Work out the finished part from the listing and answer in its coordinate system (mm). Face numbers are marked on the shaded views. A direction names the side the tool comes from. Round coordinates to 2 decimals unless told otherwise and drop trailing zeros. Order: outer loops, then holes, each group sorted by start corner. A loop starts at its lowest first (then second) coordinate and runs counter-clockwise, first axis right, second up. Notation, with made-up numbers: (12, 56) - (68, 56) arc R16 ccw to (68, 84) - close; hole circle Ø6 at (55.25, -28.75). An arc over 180 degrees is marked (long way). Use one line per item in the form item = value. Start each with the question number.
Q1. The part is cut by section D-D on z = -8.5. Determine the outline of the cut face in (x, y).
Q2. The part is cut by section C-C on x = 33.5. Determine the outline of the cut face in (y, z).
Q3. The part is cut by section B-B on z = -27.5. Determine the outline of the cut face in (x, y), plus the area to 3 significant figures.
Q4. The part is cut by section A-A on y = -10. Determine the outline of the cut face in (x, z), plus the area to 3 significant figures.
Q5. Given P1, Ø7.5, axis at y = 6, z = -6, coming from the +X side, flat-ended and moving along its own axis, determine where the tip first touches the part or whether it passes through.
Q6. Which of the six approach directions +Z, -Z, +X, -X, +Y, -Y give full straight-line access (tool end or side, diameter ignored) to the marked faces 1, 2 and 3?
Q7. Find the intervals of material crossed by line 1 (Y direction, x = 21.5, z = -10); line 2 (Y direction, x = 32.5, z = -27); line 3 (Y direction, x = 23.75, z = -8), in increasing order. Write a range as [from, to].
Autodesk Inventor part; units mm, degrees
ref_plane "YZ Plane" through (0, 0, 0) normal (1, 0, 0) x (0, 1, 0)
ref_plane "XZ Plane" through (0, 0, 0) normal (0, 1, 0) x (-1, 0, 0)
ref_plane "XY Plane" through (0, 0, 0) normal (0, 0, 1) x (1, 0, 0)
sketch "Sketch1" plane through (0, 0, 0) normal (0, 1, 0) x (-1, 0, 0)
  line L0 (0, 0) -> (-20, 0) construction
  line L1 (-20, 0) -> (-20, -20) construction
  line L2 (-20, -20) -> (0, -20) construction
  line L3 (0, -20) -> (0, 0) construction
  circle A0 centre (-27.5, -27.5) radius 2.6
  circle A1 centre (-27.5, -27.5) radius 9 construction
  line L4 (-20, 0) -> (-25, 0)
  line L5 (-25, 0) -> (-25, -20)
  line L6 (-20, -20) -> (-20, 0)
  arc A2 (-27.5, -20) -> (-27.5, -35) centre (-27.5, -27.5) ccw
  line L7 (-27.5, -35) -> (-20, -35)
  line L8 (-20, -20) -> (-20, -35)
  arc A3 (-27.5, -35) -> (-27.5, -20) centre (-27.5, -27.5) ccw construction
  line L9 (-27.5, -20) -> (-25, -20)
  circle A4 centre (-27.5, -27.5) radius 11
  line L10 (-34.504, -24.8178) -> (-25, 0)
  point P0 (-20, -19.4533)
  point P1 (-31.6263, -17.3032)
  dimension "d0" = 20
  dimension "d1" = 20
  dimension "d4" = 5.2
  dimension "d11" = 7.5
  dimension "d12" = 18
  dimension "d14" = 7.5
  dimension "d15" = 5
  dimension "d16" = 15
  dimension "d34" = 2
  dimension "d36" = 0
extrude "Extrusion1" add sketch "Sketch1" along normal mid plane 35 contours L6 A4 L5 L4 | L6 L8 L7 A2 L9 L5 A4
extrude "Extrusion4" cut sketch "Sketch1" along normal mid plane 27 contours A4 L10 A2 L7 L8 L6 | L6 L8 L7 A2 L9 L5 A4 | L5 L9 A2 L10 A4
sketch "Sketch3" plane through (25, -17.5, 0) normal (1, 0, 0) x (0, 0, -1)
  line L0 (35, 35) -> (0, 35) construction
  line L1 (10, 34.6833) -> (10, 0) construction
  circle A0 centre (10, 27.5) radius 3.1
  circle A1 centre (10, 7.5) radius 3.1
  circle A2 centre (10, 27.5) radius 5.5
  circle A3 centre (10, 7.5) radius 5.5
  line L2 (20, 0) -> (0, 0)
  line L3 (0, 0) -> (0, 35)
  point P0 (20, 35)
  point P1 (16.4634, 0)
  dimension "d22" = 6.2
  dimension "d23" = 6.2
  dimension "d24" = 7.5
  dimension "d41" = 11
  dimension "d42" = 11
  dimension "d43" = 7.5
  dimension "d50" = 10
extrude "Extrusion3" cut sketch "Sketch3" against normal up to surface (5 mm away) contours A0 | A1
extrude "Extrusion5" add sketch "Sketch1" along normal mid plane 35 contours L5 A4 L10 | L5 L9 A2 L10 A4
extrude "Extrusion6" cut sketch "Sketch1" along normal mid plane 27 contours L5 A4 L10 | L5 L9 A2 L10 A4
extrude "Extrusion7" cut sketch "Sketch3" along normal up to next
fillet "Fillet3" radius 2 1 edges at (25, 0, -16.7879)
properties part number "IdlerPulley Holder"
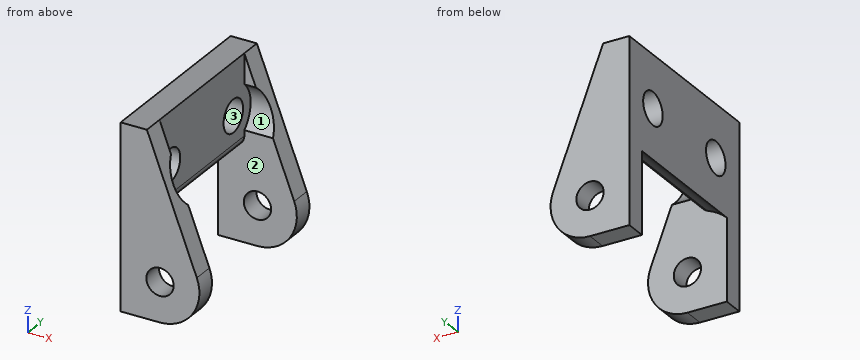
Found:
q1.outline = (20, -17.5) - (28.26, -17.5) - (28.26, -15.29) - (25, -15.29) - (25, -12.71) - (20, -12.71) - close; (20, -7.29) - (25, -7.29) - (25, 7.29) - (20, 7.29) - close; (20, 12.71) - (25, 12.71) - (25, 15.29) - (28.26, 15.29) - (28.26, 17.5) - (20, 17.5) - close
q2.outline = (-17.5, -32) - (-13.5, -32) - (-13.5, -22.2) - (-17.5, -22.2) - close; (13.5, -32) - (17.5, -32) - (17.5, -22.2) - (13.5, -22.2) - close
q3.outline = (20, -17.5) - (24.9, -17.5) - (24.9, -13.5) - (20, -13.5) - close; (20, 13.5) - (24.9, 13.5) - (24.9, 17.5) - (20, 17.5) - close; (30.1, -17.5) - (35, -17.5) - (35, -13.5) - (30.1, -13.5) - close; (30.1, 13.5) - (35, 13.5) - (35, 17.5) - (30.1, 17.5) - close
q3.area = 78.4 mm²
q4.outline = (20, -19.45) arc R11 cw to (23.69, -17.18) arc R2 ccw to (25, -15.3) - (25, -13.1) - (20, -13.1) - close; (20, -6.9) - (25, -6.9) - (25, 0) - (20, 0) - close
q4.area = 57.8 mm²
q5.P1 = 25
q6.face_1 = +X
q6.face_2 = -Z, +X
q6.face_3 = +X, -X
q7.line_1 = [-17.5, -13.1], [-6.9, 6.9], [13.1, 17.5]
q7.line_2 = [-17.5, -13.5], [13.5, 17.5]
q7.line_3 = [-17.5, -12.37], [-7.63, 7.63], [12.37, 17.5]
